from build123d import *

# Parameters (mm, degrees)
F0_W      = 120
F0_H      = 50
F1_DEPTH  = 2
F2_W      = 15
F2_H      = 10
F3_DEPTH  = 25
F4_W      = 15
F4_H      = 10
F5_DEPTH  = 12.5
F6_W      = 15
F6_H      = 10
F7_DEPTH  = 25
F8_W      = 15
F8_H      = 10
F9_DEPTH  = 25
F10_W     = 90
F10_H     = 2.5
F11_DEPTH = 10
F12_W     = 90
F12_H     = 2.5
F13_DEPTH = 10
F14_R     = 5
F15_R     = 5
F16_R     = 10
F17_R     = 10
F18_R     = 1.5
F19_DEPTH = 37.001
F20_DEPTH = 25


with BuildPart() as f1:
    # F0 (on Top) → F1 (new body)
    with BuildSketch(Plane.XY):
        Rectangle(F0_W, F0_H)
    extrude(amount=F1_DEPTH)

    # F2 (on face) → F3 (cut)
    with BuildSketch(Plane.XY.offset(2)):
        with Locations((37.5, -20)):
            Rectangle(F2_W, F2_H)
    extrude(amount=-F3_DEPTH, mode=Mode.SUBTRACT)

    # F4 (on face) → F5 (cut, symmetric)
    with BuildSketch(Plane.XY.offset(2)):
        with Locations((37.5, 20)):
            Rectangle(F4_W, F4_H)
    extrude(amount=F5_DEPTH, both=True, mode=Mode.SUBTRACT)

    # F6 (on face) → F7 (cut)
    with BuildSketch(Plane.XY.offset(2)):
        with Locations((-37.5, 20)):
            Rectangle(F6_W, F6_H)
    extrude(amount=-F7_DEPTH, mode=Mode.SUBTRACT)

    # F8 (on face) → F9 (cut)
    with BuildSketch(Plane.XY.offset(2)):
        with Locations((-37.5, -20)):
            Rectangle(F8_W, F8_H)
    extrude(amount=-F9_DEPTH, mode=Mode.SUBTRACT)

    # F10 (on face) → F11 (join)
    with BuildSketch(Plane.XY.offset(2)):
        with Locations((0, -10.75)):
            Rectangle(F10_W, F10_H)
    extrude(amount=F11_DEPTH)

    # F12 (on face) → F13 (join)
    with BuildSketch(Plane.XY.offset(2)):
        with Locations((0, 10.75)):
            Rectangle(F12_W, F12_H)
    extrude(amount=F13_DEPTH)

    # F14
    f14_edges = [f1.edges().sort_by_distance(p)[0] for p in [
        (-45, -10.75, 12),
    ]]
    fillet(f14_edges, radius=F14_R)

    # F15
    f15_edges = [f1.edges().sort_by_distance(p)[0] for p in [
        (45, 10.75, 12),
        (-45, 10.75, 12),
        (45, -10.75, 12),
    ]]
    fillet(f15_edges, radius=F15_R)

    # F16
    f16_edges = [f1.edges().sort_by_distance(p)[0] for p in [
        (60, -25, 1),
        (60, 25, 1),
    ]]
    fillet(f16_edges, radius=F16_R)

    # F17
    f17_edges = [f1.edges().sort_by_distance(p)[0] for p in [
        (-60, -25, 1),
        (-60, 25, 1),
    ]]
    fillet(f17_edges, radius=F17_R)

    # F18 (on face) → F19 (cut, through all)
    with BuildSketch(Plane.XZ.offset(12)):
        with Locations((-37.5, 6)):
            Circle(F18_R)
    extrude(amount=-F19_DEPTH, mode=Mode.SUBTRACT)

    # F18 (on face) → F20 (cut)
    with BuildSketch(Plane.XZ.offset(12)):
        with Locations((-37.5, 6)):
            Circle(F18_R)
        with Locations((37.5, 6)):
            Circle(F18_R)
    extrude(amount=-F20_DEPTH, mode=Mode.SUBTRACT)


solid = f1.part
Design review of the part built by this model. Coordinates are the model's own, in mm. A direction names the side the tool comes from. Coordinates: 2 decimals unless noted, no trailing zeros. Order: outer loops, then holes, each group sorted by start corner. A loop starts at its lowest first (then second) coordinate and runs counter-clockwise, first axis right, second up. Notation, with made-up numbers: (61, -11) -> (119, -11) arc R24 cw to (119, 7) -> close; hole circle Ø9 at (56.25, 10). An arc over 180 degrees is marked (long way). Use one line per item in the form item = value. Start each with the question number.
(1) Insertion check: pin 1 (1 mm diameter, centred on x = -38, z = 1, fed in from +Y); pin 2 (2 mm diameter, centred on y = 11, z = 5.5, fed in from -X); pin 3 (1.6 mm diameter, centred on y = -17.5, z = 1, fed in from +X); pin 4 (4 mm diameter, centred on x = -1, y = 12.5, fed in from +Z). Each pin has a flat end and moves straight along its axis. Give the tip position at first contact, or say it passes through.
(2) For probe 1 along Z at (x, y) = (-37.5, 10.2); probe 2 along Y at (x, z) = (4, 8); probe 3 along Z at (x, y) = (-37, -10), list the stretches that pass through material, from the lowest coordinate up.
(3) Add section B-B on y = 18. State the section outline as (x, z) points, plus the area to 3 significant figures.
(4) For faces 4 (the flat face through (30, -20, 1)), 5 (the flat face through (-1, -9.5, 7)), 6 (the flat face through (-38, 15, 1)), list the 3-axis set-ups (+Z, -Z, +X, -X, +Y, -Y) from which the entire face can be reached by the end or side of a thin tool; tool diameter is ignored.
(5) Add section C-C on z = 9. State the section outline as (x, y) points, plus the area to 3 significant figures.
(6) Add section A-A on x = -37.5. State the section outline as (y, z) points.
(7) Add section D-D on x = 17. State the section outline as (y, z) points.
(8) The part is to be moulded in two halves that separate along X. For faces 1 (the flat face through (-1, -12, 7)), 2 (the flat face through (-30, 20, 1)), 3 (the flat face through (-45, -11, 4)), say which applies: +X half, -X half, draft (parallel to the pull), parting line (faces both ways), or undercut.
Answer block:
q1.pin_1 = 15
q1.pin_2 = -45
q1.pin_3 = 59.85
q1.pin_4 = 12
q2.probe_1 = 0 to 4.5, 7.5 to 12
q2.probe_2 = -12 to -9.5, 9.5 to 12
q2.probe_3 = 0 to 4.59, 7.41 to 12
q3.outline = (-59.54, 0) -> (-45, 0) -> (-45, 2) -> (-59.54, 2) -> close; (-30, 0) -> (30, 0) -> (30, 2) -> (-30, 2) -> close; (45, 0) -> (59.54, 0) -> (59.54, 2) -> (45, 2) -> close
q3.area = 178 mm²
q4.face_4 = +Z, -Z, -Y
q4.face_5 = +Z, +X, -X
q4.face_6 = +Z, -Z, +Y
q5.outline = (-44.58, -12) -> (44.58, -12) -> (44.58, -9.5) -> (-44.58, -9.5) -> close; (-44.58, 9.5) -> (44.58, 9.5) -> (44.58, 12) -> (-44.58, 12) -> close
q5.area = 446 mm²
q6.outline = (-15, 0) -> (15, 0) -> (15, 2) -> (12, 2) -> (12, 4.5) -> (9.5, 4.5) -> (9.5, 2) -> (-9.5, 2) -> (-9.5, 4.5) -> (-12, 4.5) -> (-12, 2) -> (-15, 2) -> close; (-12, 7.5) -> (-9.5, 7.5) -> (-9.5, 12) -> (-12, 12) -> close; (9.5, 7.5) -> (12, 7.5) -> (12, 12) -> (9.5, 12) -> close
q7.outline = (-25, 0) -> (25, 0) -> (25, 2) -> (12, 2) -> (12, 12) -> (9.5, 12) -> (9.5, 2) -> (-9.5, 2) -> (-9.5, 12) -> (-12, 12) -> (-12, 2) -> (-25, 2) -> close
q8.face_1 = draft
q8.face_2 = undercut
q8.face_3 = -X half
